```python
from build123d import *

# Parameters (mm, degrees)
SKETCH1_W                = 44.45
SKETCH1_H                = 6.35
BOSS_EXTRUDE1_DEPTH      = 50.8
BOSS_EXTRUDE2_DEPTH      = 6.35
BOSS_EXTRUDE2_DEPTH_BACK = 50.8
SKETCH2_W                = 16.933333333
SKETCH2_H                = 6.35
SKETCH4_W                = 12.7
SKETCH4_H                = 6.35
BOSS_EXTRUDE4_DEPTH      = 6.35
CUT_EXTRUDE1_DEPTH       = 59.630138368


with BuildPart() as part:
    # Sketch1 → Boss-Extrude1 (new body)
    with BuildSketch(Plane.XY):
        with Locations((0, -17.4625)):
            Rectangle(SKETCH1_W, SKETCH1_H)
    extrude(amount=BOSS_EXTRUDE1_DEPTH)

    # Sketch2 → Boss-Extrude2 (add, two sides: drawn at the far end of the back side and taken through both)
    with BuildSketch(Plane.ZY.offset(22.225).offset(-BOSS_EXTRUDE2_DEPTH_BACK)):
        with Locations((42.333333334, -17.4625)):
            Rectangle(SKETCH2_W, SKETCH2_H)
        with Locations((8.466666667, -17.4625)):
            Rectangle(SKETCH2_W, SKETCH2_H)
    extrude(amount=BOSS_EXTRUDE2_DEPTH + BOSS_EXTRUDE2_DEPTH_BACK)

    # Sketch4 → Boss-Extrude4 (add)
    with BuildSketch(Plane(origin=(0, 0, 0), x_dir=(-1, 0, 0), z_dir=(0, 0, -1))):
        with Locations((22.225, -17.4625)):
            Rectangle(SKETCH4_W, SKETCH4_H)
        with Locations((-22.225, -17.4625)):
            Rectangle(SKETCH4_W, SKETCH4_H)
    extrude(amount=BOSS_EXTRUDE4_DEPTH)

    # Sketch5 → Cut-Extrude1 (cut, through all)
    with BuildSketch(Plane(origin=(0, -20.6375, 0), x_dir=(-1, 0, 0), z_dir=(0, -1, 0))):
        Polygon((2.0955, 0), (-2.0955, 0), (-2.0955, -8.763), (-3.429, -8.763), (-3.429, -11.303), (-2.0955, -11.303), (-2.0955, -14.605), (2.0955, -14.605), (2.0955, -11.303), (3.429, -11.303), (3.429, -8.763), (2.0955, -8.763), align=None)
    extrude(amount=-CUT_EXTRUDE1_DEPTH, mode=Mode.SUBTRACT)


solid = part.part
```
Design review of the part built by this model. Coordinates are the model's own, in mm. A direction names the side the tool comes from. Round coordinates to 2 decimals unless told otherwise and drop trailing zeros. Order: outer loops, then holes, each group sorted by start corner. A loop starts at its lowest first (then second) coordinate and runs counter-clockwise, first axis right, second up. Notation, with made-up numbers: (46.5, 67) - (82.5, 67) arc R17 cw to (82.5, 86) - close; hole circle Ø10 at (-37, 8). An arc over 180 degrees is marked (long way). One line per question, with ' | ' between items.
Item 1: For P1, Ø1.1, axis at x = -3, y = -18.5, coming from the -Z side; P2, Ø2, axis at y = -16, z = 19, coming from the +X side (3 decimals), all flat-tipped, find the tip position at first contact; note any pin that passes through.
Checks:
P1: z = 0 | P2: x = 22.225
Item 2: Take a section at C-C, the plane x = 9. Write out the cut boundary in (y, z), then the cut area to 3 significant figures.
Checks:
outline: (-20.64, 0) - (-14.29, 0) - (-14.29, 50.8) - (-20.64, 50.8) - close | area: 323 mm²
Item 3: Take a section at A-A, the plane z = 7. Write out the cut boundary in (x, y) (1 decimal).
Checks:
outline: (-28.6, -20.6) - (-2.1, -20.6) - (-2.1, -14.3) - (-28.6, -14.3) - close; (2.1, -20.6) - (28.6, -20.6) - (28.6, -14.3) - (2.1, -14.3) - close
Item 4: Take a section at D-D, the plane z = 28.5. Write out the cut boundary in (x, y) (1 decimal), then the cut area to 3 significant figures.
Checks:
outline: (-22.2, -20.6) - (22.2, -20.6) - (22.2, -14.3) - (-22.2, -14.3) - close | area: 282 mm²
Item 5: Wall thickness on line 1 (X direction, y = -18, z = 2) (1 decimal); line 2 (X direction, y = -15.25, z = -0.5) (3 decimals); line 3 (Z direction, x = 4, y = -15.5): over which ranges is each line inside the solid? List them lowest first. Write a range as [from, to].
Checks:
line 1: [-28.6, -2.1], [2.1, 28.6] | line 2: [-28.575, -15.875], [15.875, 28.575] | line 3: [0, 50.8]
Item 6: Draft analysis for pull direction Z (two halves, no side actions). For faces 4 (the face through (0, -18, 14.605)), 5 (the face through (2.096, -18, 4)), 6 (the face through (25, -18, 16.933)), state which applies: +Z half, -Z half, draft (parallel to the pull), parting line (faces both ways), or undercut.
Checks:
face 4: -Z half | face 5: draft | face 6: undercut
Item 7: Machinability: for faces 1 (the face through (-3.429, -18, 10)), 2 (the face through (-2.096, -18, 13)), 3 (the face through (25, -18, 33.867)), which of the approach directions +Z, -Z, +X, -X, +Y, -Y give a long, thin tool a straight path to every point of the face, cutting with its end or side? Answer none if there is none.
Checks:
face 1: +Y, -Y | face 2: -Z, +Y, -Y | face 3: +X, +Y, -Y
